Geometry: final body of the model. Coordinates: model frame, mm. A direction names the side the tool comes from. Give positions to 0.01 mm unless a question says otherwise; leave off trailing zeros. Write each loop counter-clockwise with the first axis right and the second up, starting at its lowest first coordinate (ties: lowest second). Pieces come first, ordered by that corner, then holes.
Q1. Line query: L1, parallel to Z at x = -7.75, y = 19.5; L2, parallel to Z at x = 3.75, y = 18; L3, parallel to X at y = 15.5, z = 3. Output: solid intervals per line, ascending.
Q2. Cut plane A-A on x = 0. Return the cut outline in (y, z).
Q3. Cut plane B-B on z = 6. Return the cut outline in (x, y), plus the area to 3 significant figures.
Q4. Draft query along X for faces 3 (the face through (6.5, 21.24, 3.1)), 4 (the face through (-6.034, 10.769, -3.549)), 5 (the face through (-14.985, 10.471, -0.66)). Return one class per face: pulls with the +X half, pulls with the -X half, needs draft (parallel to the pull), parting line crosses it, or undercut.
Q5. Pin query (flat end, axial travel): pin 1 (1 mm diameter, centred on x = 11.5, y = 4.5, fed in from -Z); pin 2 (1 mm diameter, centred on y = 15.5, z = -11.5, fed in from +X); pin 3 (5 mm diameter, centred on x = -10.5, y = 6, fed in from -Z); pin 4 (3 mm diameter, centred on x = -1, z = 4.5, fed in from +Y). Return the tip coordinate at first contact, or that it passes through.
Q6. Reachability of faces 1 (the face through (6.09, 10.77, -3.45)), 2 (the face through (6.5, 0, 3.1)) from +Z, -Z, +X, -X, +Y, -Y: full face, straight path, thin tool, end or side. Return the list, or none.
Q7. Cut plane C-C on y = 11.75. Return the cut outline in (x, z).
Q8. Cut plane D-D on x = -9. Return the cut outline in (y, z).
```python
from build123d import *

# Parameters (mm, degrees)
SKETCH1_R               = 15
BOSS_EXTRUDE1_DEPTH     = 21.24
CUT_EXTRUDE1_DEPTH      = 26
CUT_EXTRUDE1_DEPTH_BACK = 32


with BuildPart() as part:
    # Sketch1 → Boss-Extrude1 (new body)
    with BuildSketch(Plane(origin=(0, 0, 0), x_dir=(1, 0, 0), z_dir=(0, 1, 0))):
        Circle(SKETCH1_R)
    extrude(amount=BOSS_EXTRUDE1_DEPTH)

    # Sketch3 → Cut-Extrude1 (cut, two sides)
    with BuildSketch(Plane(origin=(0, 21.24, 0), x_dir=(1, 0, 0), z_dir=(0, 1, 0))) as cut_extrude1_sk:
        Polygon((8.082903769, 0), (4.041451884, 7), (-4.041451884, 7), (-8.082903769, 0), (-4.041451884, -7), (4.041451884, -7), align=None)
    extrude(amount=CUT_EXTRUDE1_DEPTH, mode=Mode.SUBTRACT)
    extrude(cut_extrude1_sk.sketch, amount=-CUT_EXTRUDE1_DEPTH_BACK, mode=Mode.SUBTRACT)


solid = part.part
```
Data:
1. L1: z = -12.84 to -0.58, 0.58 to 12.84
1. L2: z = -14.52 to -7, 7 to 14.52
1. L3: x = -14.7 to -6.35, 6.35 to 14.7
2. outline: (0, -15) - (21.24, -15) - (21.24, -7) - (0, -7) - close; (0, 7) - (21.24, 7) - (21.24, 15) - (0, 15) - close
3. outline: (-13.75, 0) - (-4.62, 0) - (-4.62, 21.24) - (-13.75, 21.24) - close; (4.62, 0) - (13.75, 0) - (13.75, 21.24) - (4.62, 21.24) - close
3. area: 388 mm2
4. face 3: needs draft
4. face 4: undercut
4. face 5: parting line crosses it
5. pin 1: stops at z = -10.2
5. pin 2: stops at x = 10.2
5. pin 3: stops at z = -12.69
5. pin 4: passes through
6. face 1: +Y, -Y
6. face 2: +Z, -Z, +X, -X, -Y
7. outline: circle Ø30 at (0, 0); hole (-8.08, 0) - (-4.04, -7) - (4.04, -7) - (8.08, 0) - (4.04, 7) - (-4.04, 7) - close
8. outline: (0, -12) - (21.24, -12) - (21.24, 12) - (0, 12) - close
